Check sheet for the modelled part. Datum: model origin and axes. Units: mm. Face numbers are marked on the shaded views. A direction names the side the tool comes from. Give positions to 0.01 mm unless a question says otherwise; leave off trailing zeros. Loops run counter-clockwise (first coordinate to the right, second up) from the corner with the lowest first, then second, coordinate; pieces in that order, holes last. Notation, with made-up numbers: (23, 89.25) - (80, 89.25) arc R9 cw to (80, 95.25) - close; hole circle Ø4 at (10, 34). An arc over 180 degrees is marked (long way). Answer in a Markdown table with one row per item. Add a question column.
(1) Draft check along X on the marked faces 1, 2 and 3. Enter one of: released by +X, released by -X, zero draft, split by the parting line, or undercut.
(2) Sectioned sample at B-B on y = 2.5. Enter the section's corners in (x, z).
(3) Thickness scan on L1, parallel to X at y = 16, z = 16; L2, parallel to X at y = 1.5, z = 16.75; L3, parallel to Z at x = -24, y = 8. Record the ranges inside material, lowest first.
(4) Sectioned sample at A-A on z = 10. Enter the section's corners in (x, y).
(5) Go/stop test with a flat-tipped pin: P1, Ø6, axis at y = -9, z = 10.5, coming from the -X side. Record where the tip stops, or that it passes through.
(6) Set-up check for the marked faces 4 and 5: record each of +Z, -Z, +X, -X, +Y, -Y from which the full face is reachable in a straight line by a thin tool's end or side.
(7) Sectioned sample at C-C on z = 13.5. Enter the section's corners in (x, y).
(8) Sectioned sample at D-D on y = 10. Enter the section's corners in (x, z).
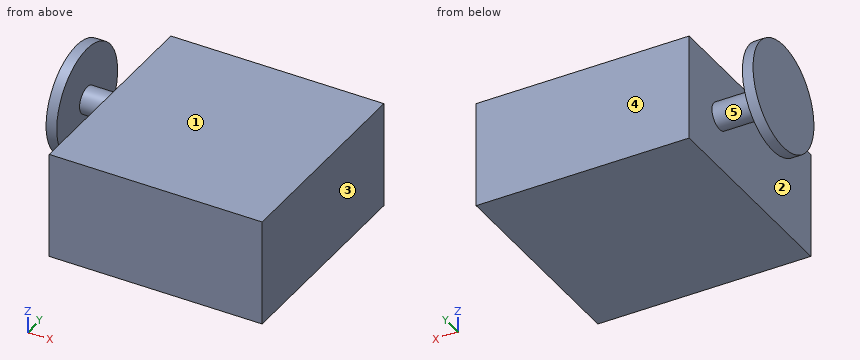
from build123d import *

# Parameters (mm, degrees)
SKETCH_1_W      = 40
SKETCH_1_H      = 40
EXTRUDE_1_DEPTH = 20
SKETCH_2_R      = 2.5
EXTRUDE_2_DEPTH = 10
SKETCH_3_R      = 10
EXTRUDE_3_DEPTH = 2


with BuildPart() as part:
    # 草图1 → 凸台-拉伸1 (new body)
    with BuildSketch(Plane.XY):
        Rectangle(SKETCH_1_W, SKETCH_1_H)
    extrude(amount=EXTRUDE_1_DEPTH)

    # 草图2 → 凸台-拉伸2 (add)
    with BuildSketch(Plane.ZY.offset(20)):
        with Locations(Location((10, 10, 0), (0, 0, 180))):
            Circle(SKETCH_2_R)
    extrude(amount=EXTRUDE_2_DEPTH)

    # 草图3 → 凸台-拉伸3 (add)
    with BuildSketch(Plane.ZY.offset(30)):
        with Locations((10, 10)):
            Circle(SKETCH_3_R)
    extrude(amount=EXTRUDE_3_DEPTH)


solid = part.part
Reply:
| question | item | result |
|---|---|---|
| 1 | face 1 | zero draft |
| 1 | face 2 | undercut |
| 1 | face 3 | released by +X |
| 2 | outline | (-32, 3.39) - (-30, 3.39) - (-30, 16.61) - (-32, 16.61) - close; (-20, 0) - (20, 0) - (20, 20) - (-20, 20) - close |
| 3 | L1 | -32 to -30, -20 to 20 |
| 3 | L2 | -20 to 20 |
| 3 | L3 | 8.5 to 11.5 |
| 4 | outline | (-32, 0) - (-30, 0) - (-30, 7.5) - (-20, 7.5) - (-20, -20) - (20, -20) - (20, 20) - (-20, 20) - (-20, 12.5) - (-30, 12.5) - (-30, 20) - (-32, 20) - close |
| 5 | P1 | x = -20 |
| 6 | face 4 | +Z, -Z, +X, -X, +Y |
| 6 | face 5 | none |
| 7 | outline | (-32, 0.63) - (-30, 0.63) - (-30, 19.37) - (-32, 19.37) - close; (-20, -20) - (20, -20) - (20, 20) - (-20, 20) - close |
| 8 | outline | (-32, 0) - (-30, 0) - (-30, 7.5) - (-20, 7.5) - (-20, 0) - (20, 0) - (20, 20) - (-20, 20) - (-20, 12.5) - (-30, 12.5) - (-30, 20) - (-32, 20) - close |
